Geometry: final body of the model. Coordinates: model frame, mm. A direction names the side the tool comes from. Coordinates: 2 decimals unless noted, no trailing zeros. Loops run counter-clockwise (first coordinate to the right, second up) from the corner with the lowest first, then second, coordinate; pieces in that order, holes last. Notation, with made-up numbers: (69.25, 1.5) -> (119.25, 1.5) arc R16 ccw to (119.25, 11.5) -> close; hole circle Ø7 at (-28, 50.5). An arc over 180 degrees is marked (long way). One line per item, written item: value. Start each with the question number.
from build123d import *

# Parameters (mm, degrees)
CUT_EXTRUDE1_DEPTH      = 9
SKETCH3_R               = 2.5
CUT_EXTRUDE2_DEPTH      = 2.5
SKETCH4_R               = 4
BOSS_EXTRUDE1_DEPTH     = 7
SKETCH5_R               = 1.25
CUT_EXTRUDE3_DEPTH      = 11
CUT_EXTRUDE3_DEPTH_BACK = 11


with BuildPart() as part:
    # Sketch1 → Revolve1 (revolve)
    with BuildSketch(Plane.XY):
        Polygon((20, 0), (-20, 0), (-20, 10), (-16.5, 5), (-3.5, 5), (0, 10), (3.5, 5), (16.5, 5), (20, 10), align=None)
    revolve(axis=Axis((20, 0, 0), (-1, 0, 0)))

    # Sketch2 → Cut-Extrude1 (cut)
    with BuildSketch(Plane.ZY.offset(20)):
        with BuildLine():
            ThreePointArc((1.5, 2), (0, 2.5), (-1.5, 2))
            Line((-1.5, 2), (-1.5, -2))
            ThreePointArc((-1.5, -2), (0, -2.5), (1.5, -2))
            Line((1.5, -2), (1.5, 2))
        make_face()
    extrude(amount=-CUT_EXTRUDE1_DEPTH, mode=Mode.SUBTRACT)

    # Sketch3 → Cut-Extrude2 (cut)
    with BuildSketch(Plane.ZY.offset(20)):
        Circle(SKETCH3_R)
    extrude(amount=-CUT_EXTRUDE2_DEPTH, mode=Mode.SUBTRACT)

    # Sketch4 → Boss-Extrude1 (add)
    with BuildSketch(Plane(origin=(20, 0, 0), x_dir=(0, 0, -1), z_dir=(1, 0, 0))):
        Circle(SKETCH4_R)
    extrude(amount=BOSS_EXTRUDE1_DEPTH)

    # Sketch5 → Cut-Extrude3 (cut, two sides)
    with BuildSketch(Plane(origin=(0, 0, 0), x_dir=(1, 0, 0), z_dir=(0, 1, 0))) as cut_extrude3_sk:
        with Locations((-7, 0)):
            Circle(SKETCH5_R)
        with Locations((7, 0)):
            Circle(SKETCH5_R)
    extrude(amount=CUT_EXTRUDE3_DEPTH, mode=Mode.SUBTRACT)
    extrude(cut_extrude3_sk.sketch, amount=-CUT_EXTRUDE3_DEPTH_BACK, mode=Mode.SUBTRACT)


solid = part.part
1. Pin query (flat end, axial travel): pin 1 Ø1.5 at (x, z) = (-7, 0) entering from +Y; pin 2 Ø4 at (x, z) = (-7, 0) entering from -Y; pin 3 Ø1.5 at (y, z) = (-1, -0.5) entering from -X; pin 4 Ø3 at (x, y) = (-15.5, -1) entering from +Z. Return the tip coordinate at first contact, or that it passes through.
2. Draft query along Z for faces 1 (the face through (-20, -2, 2)), 2 (the face through (-3.28, 5.07, -1.6)), 3 (the face through (-11, 0, 0)). Return one class per face: released by +Z, released by -Z, zero draft, split by the parting line, or undercut.
3. Section A-A on z = 0. Count the separate pieces of the cut face and the enclosed holes in it, plus the area to 3 significant figures.
4. Set-up query: faces 4 (the face through (-16.67, -1.14, 5.12)), 5 (the face through (27, 0, 0)), 6 (the face through (23.451, -3.905, 0.867)), 7 (the face through (-17.5, 0, -2)). Return all of +Z, -Z, +X, -X, +Y, -Y with unobstructed straight access to the full face (end or side cutting, diameter ignored); none if empty.
5. Section B-B on x = -11.5. Return the cut outline in (y, z).
6. Line query: L1, parallel to X at y = -8.5, z = 1.5; L2, parallel to X at y = -1.1, z = 0; L3, parallel to Z at x = -16.25, y = 0. Output: solid intervals per line, ascending. Write a range as [from, to].
7. Section C-C on x = 7. Return the cut outline in (y, z).
Checks:
1. pin 1: through
1. pin 2: y = -5
1. pin 3: x = -11
1. pin 4: z = 5.64
2. face 1: zero draft
2. face 2: split by the parting line
2. face 3: undercut
3. separate pieces: 3
3. enclosed holes: 0
3. area: 431 mm²
4. face 4: none
4. face 5: +Z, -Z, +X, +Y, -Y
4. face 6: +X
4. face 7: -X
5. outline: circle Ø10 at (0, 0); hole (-2, -1.5) -> (2, -1.5) arc R2.5 ccw to (2, 1.5) -> (-2, 1.5) arc R2.5 ccw to start
6. L1: [-20, -19.04], [-0.96, 0.96], [19.04, 20]
6. L2: [-11, -8.25], [-5.75, 5.75], [8.25, 27]
6. L3: [-5, -1.5], [1.5, 5]
7. outline: (-4.84, -1.25) arc R5 ccw to (4.84, -1.25) -> close; (-4.84, 1.25) -> (4.84, 1.25) arc R5 ccw to start
